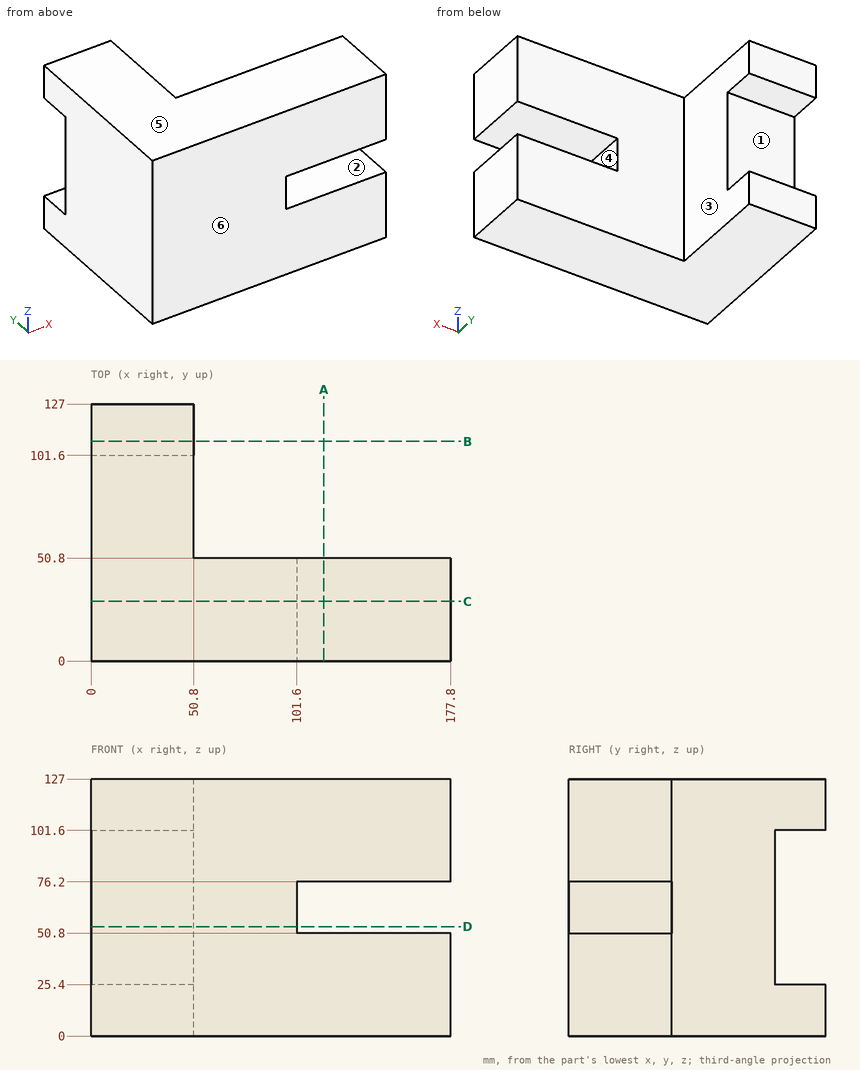
Could you check a few things on this drawing? It's one solid part, dimensions in mm from its lowest x, y, z. A direction names the side the tool comes from. Give positions to 0.01 mm unless a question says otherwise; leave off trailing zeros. Loops run counter-clockwise (first coordinate to the right, second up) from the corner with the lowest first, then second, coordinate; pieces in that order, holes last. Notation, with made-up numbers: M 64,-1 L 76,-1 A31 ccw 76,36 Z; hole C -38.75,33 d4. An arc over 180 degrees is marked long. Return JSON: item names as keys, results as strings.
Item 1: Imagine slicing it at A-A on x = 115. List the corners of the cut face in (y, z) for me, then the cut area to 3 significant figures.
A:
{"outline": "M 0,0 L 50.8,0 L 50.8,50.8 L 0,50.8 Z; M 0,76.2 L 50.8,76.2 L 50.8,127 L 0,127 Z", "area": "5,160 mm^2"}
Item 2: Please list where these lines run through material, in increasing order: line 1 (Y direction, x = 72, z = 29); line 2 (Y direction, x = 10, z = 47.5).
A:
{"line 1": "y = 0 to 50.8", "line 2": "y = 0 to 101.6"}
Item 3: Imagine slicing it at D-D on z = 54. List the corners of the cut face in (x, y) for me, then the cut area to 3 significant figures.
A:
{"outline": "M 0,0 L 101.6,0 L 101.6,50.8 L 50.8,50.8 L 50.8,101.6 L 0,101.6 Z", "area": "7,740 mm^2"}
Item 4: I'm going to push flat-ended pins straight in: pin 1 Ø3 at (x, z) = (64, 82.5) entering from -Y; pin 2 Ø12 at (y, z) = (83.5, 96) entering from +X; pin 3 Ø1.5 at (x, z) = (56.5, 66) entering from +Y. Where does each tip first touch, or does it pass through?
A:
{"pin 1": "stops at y = 0", "pin 2": "stops at x = 50.8", "pin 3": "stops at y = 50.8"}
Item 5: Imagine slicing it at B-B on y = 108.5. List the corners of the cut face in (x, z) for me.
A:
{"outline": "M 0,0 L 50.8,0 L 50.8,25.4 L 0,25.4 Z; M 0,101.6 L 50.8,101.6 L 50.8,127 L 0,127 Z"}
Item 6: On a 3-axis mill with a long thin cutter (end or side, diameter ignored), from which of +Z, -Z, +X, -X, +Y, -Y can I reach the whole of each face in a straight line? I mean the marked faces 1, 2 and 3. Say none if no direction works.
A:
{"face 1": "+X, -X, +Y", "face 2": "+X, +Y, -Y", "face 3": "+Z, -Z, +X, +Y"}
Item 7: Thinking about a two-plate mould opening in Z: for the marked faces 4, 5 and 6, which applies, released by +Z, released by -Z, zero draft, split by the parting line, or undercut?
A:
{"face 4": "undercut", "face 5": "released by +Z", "face 6": "zero draft"}
Item 8: Imagine slicing it at C-C on y = 29.5. List the corners of the cut face in (x, z) for me.
A:
{"outline": "M 0,0 L 177.8,0 L 177.8,50.8 L 101.6,50.8 L 101.6,76.2 L 177.8,76.2 L 177.8,127 L 0,127 Z"}
